For this review, take the finished solid that the model builds, in its own axes (mm). Face numbers are marked on the shaded views. A direction names the side the tool comes from. Round coordinates to 2 decimals unless told otherwise and drop trailing zeros. Order: outer loops, then holes, each group sorted by start corner. A loop starts at its lowest first (then second) coordinate and runs counter-clockwise, first axis right, second up. Notation, with made-up numbers: M -28,38 L 17,38 A15 ccw 17,62 Z; hole C -27,8 d7. An arc over 180 degrees is marked long. Use a Markdown table: item, result.
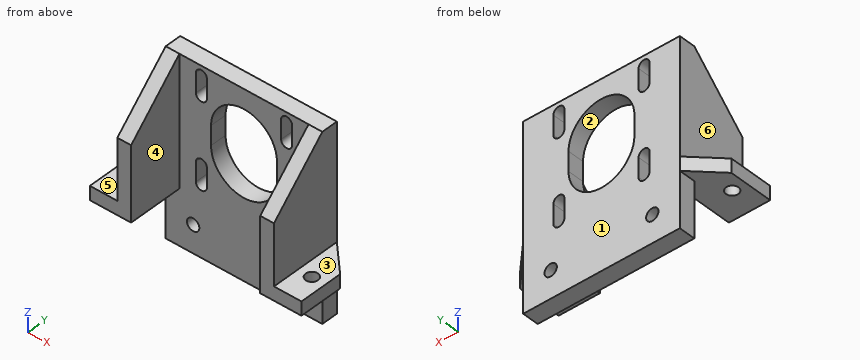
from build123d import *

# Parameters (mm, degrees)
SKETCH1_W           = 57
SKETCH1_H           = 6
BOSS_EXTRUDE1_DEPTH = 50
CUT_EXTRUDE2_DEPTH  = 10
SKETCH4_W           = 57
SKETCH4_H           = 6
BOSS_EXTRUDE2_DEPTH = 17
SKETCH6_R           = 2.25
CUT_EXTRUDE3_DEPTH  = 20
SKETCH8_W           = 5
SKETCH8_H           = 47
BOSS_EXTRUDE4_DEPTH = 20
CHAMFER1_SIZE       = 20
SKETCH9_W           = 5
SKETCH9_H           = 26
BOSS_EXTRUDE5_DEPTH = 10
SKETCH10_W          = 5
SKETCH10_H          = 26
BOSS_EXTRUDE6_DEPTH = 10
CHAMFER2_SIZE       = 10
SKETCH11_R          = 2.25
CUT_EXTRUDE4_DEPTH  = 10


with BuildPart() as part:
    # Sketch1 → Boss-Extrude1 (new body)
    with BuildSketch(Plane.XY):
        Rectangle(SKETCH1_W, SKETCH1_H)
    extrude(amount=BOSS_EXTRUDE1_DEPTH)

    # Sketch3 → Cut-Extrude2 (cut)
    with BuildSketch(Plane(origin=(0, 3, 0), x_dir=(1, 0, 0), z_dir=(0, 1, 0))):
        with BuildLine():
            Line((-13.5, -8.5), (-13.5, -15.5))
            ThreePointArc((-13.5, -15.5), (-15.5, -17.5), (-17.5, -15.5))
            Line((-17.5, -15.5), (-17.5, -8.5))
            ThreePointArc((-17.5, -8.5), (-15.5, -6.5), (-13.5, -8.5))
        make_face()
        with BuildLine():
            Line((-13.5, -39.5), (-13.5, -46.5))
            ThreePointArc((-13.5, -46.5), (-15.5, -48.5), (-17.5, -46.5))
            Line((-17.5, -46.5), (-17.5, -39.5))
            ThreePointArc((-17.5, -39.5), (-15.5, -37.5), (-13.5, -39.5))
        make_face()
        with BuildLine():
            Line((17.5, -39.5), (17.5, -46.5))
            ThreePointArc((17.5, -46.5), (15.5, -48.5), (13.5, -46.5))
            Line((13.5, -46.5), (13.5, -39.5))
            ThreePointArc((13.5, -39.5), (15.5, -37.5), (17.5, -39.5))
        make_face()
        with BuildLine():
            Line((17.5, -8.5), (17.5, -15.5))
            ThreePointArc((17.5, -15.5), (15.5, -17.5), (13.5, -15.5))
            Line((13.5, -15.5), (13.5, -8.5))
            ThreePointArc((13.5, -8.5), (15.5, -6.5), (17.5, -8.5))
        make_face()
        with BuildLine():
            Line((12, -24), (12, -31))
            ThreePointArc((12, -31), (0, -43), (-12, -31))
            Line((-12, -31), (-12, -24))
            ThreePointArc((-12, -24), (0, -12), (12, -24))
        make_face()
    extrude(amount=-CUT_EXTRUDE2_DEPTH, mode=Mode.SUBTRACT)

    # Sketch4 → Boss-Extrude2 (add)
    with BuildSketch(Plane(origin=(0, 0, 0), x_dir=(-1, 0, 0), z_dir=(0, 0, -1))):
        Rectangle(SKETCH4_W, SKETCH4_H)
    extrude(amount=BOSS_EXTRUDE2_DEPTH)

    # Sketch6 → Cut-Extrude3 (cut)
    with BuildSketch(Plane(origin=(0, 3, 0), x_dir=(1, 0, 0), z_dir=(0, 1, 0))):
        with Locations(Location((-18.5, 7, 0), (0, 0, 180))):
            Circle(SKETCH6_R)
        with Locations(Location((18.5, 7, 0), (0, 0, 180))):
            Circle(SKETCH6_R)
    extrude(amount=-CUT_EXTRUDE3_DEPTH, mode=Mode.SUBTRACT)

    # Sketch8 → Boss-Extrude4 (add)
    with BuildSketch(Plane.XZ.offset(3)):
        with Locations((-26, 26.5)):
            Rectangle(SKETCH8_W, SKETCH8_H)
        with Locations((26, 26.5)):
            Rectangle(SKETCH8_W, SKETCH8_H)
    extrude(amount=BOSS_EXTRUDE4_DEPTH)

    # Chamfer1
    chamfer1_edges = [part.edges().sort_by_distance(p)[0] for p in [
        (26, -23, 50),
        (-26, -23, 50),
    ]]
    chamfer(chamfer1_edges, length=CHAMFER1_SIZE)

    # Sketch9 → Boss-Extrude5 (add)
    with BuildSketch(Plane.ZY.offset(28.5)):
        with Locations((5.5, -10)):
            Rectangle(SKETCH9_W, SKETCH9_H)
    extrude(amount=BOSS_EXTRUDE5_DEPTH)

    # Sketch10 → Boss-Extrude6 (add)
    with BuildSketch(Plane(origin=(28.5, 0, 0), x_dir=(0, 0, -1), z_dir=(1, 0, 0))):
        with Locations((-5.5, -10)):
            Rectangle(SKETCH10_W, SKETCH10_H)
    extrude(amount=BOSS_EXTRUDE6_DEPTH)

    # Chamfer2
    chamfer2_edges = [part.edges().sort_by_distance(p)[0] for p in [
        (38.5, 3, 5.5),
        (-38.5, 3, 5.5),
    ]]
    chamfer(chamfer2_edges, length=CHAMFER2_SIZE)

    # Sketch11 → Cut-Extrude4 (cut)
    with BuildSketch(Plane.XY.offset(8)):
        with Locations((-33.5, -13)):
            Circle(SKETCH11_R)
        with Locations((33.5, -13)):
            Circle(SKETCH11_R)
    extrude(amount=-CUT_EXTRUDE4_DEPTH, mode=Mode.SUBTRACT)


solid = part.part
Q1. Machinability: for the marked faces 1, 2 and 3, which of the approach directions +Z, -Z, +X, -X, +Y, -Y give a long, thin tool a straight path to every point of the face, cutting with its end or side? Answer none if there is none.
Determined:
| item | result |
|---|---|
| face 1 | +Z, -Z, +X, -X, +Y |
| face 2 | +Y, -Y |
| face 3 | +Z, +X, +Y, -Y |
Q2. Wall thickness on line 1 along Z through (x, y) = (18.5, 1.45); line 2 along X through (y, z) = (0.5, -6); line 3 along X through (y, z) = (-1.25, 26.5): over which ranges is each line inside the solid? List them lowest first. Write a range as [from, to].
Determined:
| item | result |
|---|---|
| line 1 | z = [-17, -9.25], [-4.75, 50] |
| line 2 | x = [-28.5, -20.52], [-16.48, 16.48], [20.52, 28.5] |
| line 3 | x = [-28.5, -12], [12, 28.5] |
Q3. Add section D-D (z = 27). Write out the cut boundary in (x, y).
Determined:
| item | result |
|---|---|
| outline | M -28.5,-23 L -23.5,-23 L -23.5,-3 L -12,-3 L -12,3 L -28.5,3 Z; M 12,-3 L 23.5,-3 L 23.5,-23 L 28.5,-23 L 28.5,3 L 12,3 Z |
Q4. Add section A-A (x = 33.5). Write out the cut boundary in (y, z), then the cut area to 3 significant figures.
Determined:
| item | result |
|---|---|
| outline | M -23,3 L -15.25,3 L -15.25,8 L -23,8 Z; M -10.75,3 L -2,3 L -2,8 L -10.75,8 Z |
| area | 82.5 mm^2 |
Q5. Draft analysis for pull direction X (two halves, no side actions). For the marked faces 4, 5 and 6, state which applies: pulls with the +X half, pulls with the -X half, needs draft (parallel to the pull), parting line crosses it, or undercut.
Determined:
| item | result |
|---|---|
| face 4 | undercut |
| face 5 | needs draft |
| face 6 | pulls with the -X half |
Q6. Clearance check with flat-ended pins moving along their axes: pin 1 (1.8 mm diameter, centred on y = 0, z = -5, fed in from -X); pin 2 (6 mm diameter, centred on y = -7.5, z = 41, fed in from +X); pin 3 (3 mm diameter, centred on x = 14.5, z = 26, fed in from -Y). State where each tip first meets the part, or that it passes through.
Determined:
| item | result |
|---|---|
| pin 1 | stops at x = -28.5 |
| pin 2 | stops at x = 28.5 |
| pin 3 | stops at y = -3 |
Q7. Add section B-B (y = -18.5). Write out the cut boundary in (x, z).
Determined:
| item | result |
|---|---|
| outline | M -38.5,3 L -23.5,3 L -23.5,34.5 L -28.5,34.5 L -28.5,8 L -38.5,8 Z; M 23.5,3 L 38.5,3 L 38.5,8 L 28.5,8 L 28.5,34.5 L 23.5,34.5 Z |
Q8. Add section C-C (z = 45.5). Write out the cut boundary in (x, y), then the cut area to 3 significant figures.
Determined:
| item | result |
|---|---|
| outline | M -28.5,-7.5 L -23.5,-7.5 L -23.5,-3 L -17.5,-3 L -17.5,3 L -28.5,3 Z; M -13.5,-3 L 13.5,-3 L 13.5,3 L -13.5,3 Z; M 17.5,-3 L 23.5,-3 L 23.5,-7.5 L 28.5,-7.5 L 28.5,3 L 17.5,3 Z |
| area | 339 mm^2 |
